```python
from build123d import *

# Parameters (mm, degrees)
F1_W     = 127
F1_H     = 76.2
F2_DEPTH = 25.4
F0_R     = 38.4068488144
F4_DEPTH = 135.89


with BuildPart() as f2:
    # F1 (on Top) → F2 (new body)
    with BuildSketch(Plane.XY):
        Rectangle(F1_W, F1_H)
    extrude(amount=F2_DEPTH)


with BuildPart() as f4:
    # F0 (on Front) → F4 (new body)
    with BuildSketch(Plane.XZ):
        Circle(F0_R)
    extrude(amount=-F4_DEPTH)


solid = f4.part
```
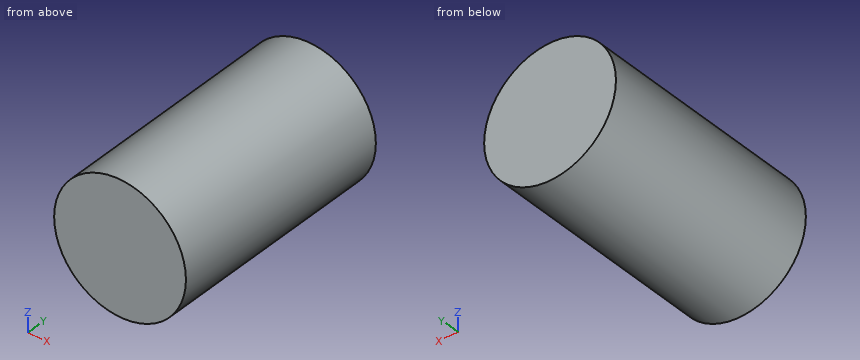
For this review, take the finished solid that the model builds, in its own axes (mm). Round coordinates to 2 decimals unless told otherwise and drop trailing zeros. Order: outer loops, then holes, each group sorted by start corner. A loop starts at its lowest first (then second) coordinate and runs counter-clockwise, first axis right, second up.
Q1. We need section B-B, the plane x = -19.5. Give the boundary of the cut face in (y, z).
Findings below:
outline: (0, -33.09) - (135.89, -33.09) - (135.89, 33.09) - (0, 33.09) - close
Q2. Insertion check: P1, Ø4, axis at x = -24.5, y = 28, coming from the +Z side; P2, Ø8, axis at y = 89.5, z = -19, coming from the -X side; P3, Ø6, axis at y = 19, z = 26, coming from the +X side. Each pin has a flat end and moves straight along its axis. Give the tip position at first contact, or say it passes through.
Findings below:
P1: stops at z = 31.13
P2: stops at x = -35.36
P3: stops at x = 30.76
Q3. We need section C-C, the plane z = -10. Give the boundary of the cut face in (x, y), plus the area to 3 significant figures.
Findings below:
outline: (-37.08, 0) - (37.08, 0) - (37.08, 135.89) - (-37.08, 135.89) - close
area: 10,100 mm2
Q4. Wall thickness on line 1 (X direction, y = 104, z = 1); line 2 (X direction, y = 84, z = 17): over which ranges is each line inside the solid? List them lowest first.
Findings below:
line 1: x = -38.39 to 38.39
line 2: x = -34.44 to 34.44
Q5. We need section A-A, the plane y = 72. Give the boundary of the cut face in (x, z).
Findings below:
outline: circle Ø76.81 at (0, 0)
